Design review of the part built by this model. Coordinates are the model's own, in mm. Round coordinates to 2 decimals unless told otherwise and drop trailing zeros. Loops run counter-clockwise (first coordinate to the right, second up) from the corner with the lowest first, then second, coordinate; pieces in that order, holes last. Notation, with made-up numbers: (46, 34.25) -> (79, 34.25) arc R12 ccw to (79, 50.25) -> close; hole circle Ø6 at (70, -15). An arc over 180 degrees is marked (long way). Use a Markdown table: item, result. Add a question column.
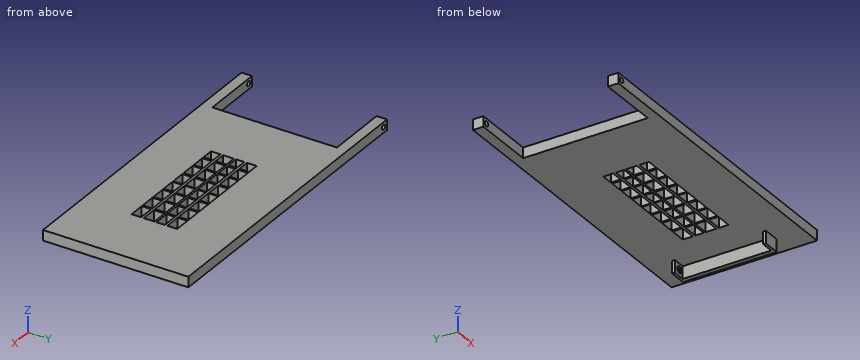
from build123d import *

# Parameters (mm, degrees)
SKETCH1_W               = 600
SKETCH1_H               = 350
BOSS_EXTRUDE1_DEPTH     = 25
SKETCH3_W               = 25
SKETCH3_H               = 25
BOSS_EXTRUDE2_DEPTH     = 150
SKETCH4_R               = 6
CUT_EXTRUDE1_DEPTH      = 370
SKETCH5_W               = 28.359872958
SKETCH5_H               = 23.680958907
SKETCH5_W_2             = 32.02157976
SKETCH5_W_3             = 34.109943658
SKETCH5_W_4             = 34.109943657
SKETCH5_W_5             = 33.413822358
SKETCH5_W_6             = 36.198307555
SKETCH5_W_7             = 38.439491831
SKETCH5_H_2             = 20.187517675
SKETCH5_H_3             = 25.762905436
SKETCH5_H_4             = 22.972002872
CUT_EXTRUDE3_DEPTH      = 30
SKETCH7_W               = 11
SKETCH7_H               = 213.013117536
BOSS_EXTRUDE4_DEPTH     = 30
SKETCH8_W               = 41.071156649
SKETCH8_H               = 6.265091692
BOSS_EXTRUDE5_DEPTH     = 30
SKETCH11_R              = 8
CUT_EXTRUDE6_DEPTH      = 217
CUT_EXTRUDE6_DEPTH_BACK = 4


with BuildPart() as part:
    # Sketch1 → Boss-Extrude1 (new body)
    with BuildSketch(Plane.XY):
        with Locations((300, 175)):
            Rectangle(SKETCH1_W, SKETCH1_H)
    extrude(amount=BOSS_EXTRUDE1_DEPTH)

    # Sketch3 → Boss-Extrude2 (add)
    with BuildSketch(Plane.ZY):
        with Locations((12.5, 12.5)):
            Rectangle(SKETCH3_W, SKETCH3_H)
        with Locations((12.5, 337.5)):
            Rectangle(SKETCH3_W, SKETCH3_H)
    extrude(amount=BOSS_EXTRUDE2_DEPTH)

    # Sketch4 → Cut-Extrude1 (cut)
    with BuildSketch(Plane.XZ):
        with Locations((-137.5, 13.055008402)):
            Circle(SKETCH4_R)
    extrude(amount=-CUT_EXTRUDE1_DEPTH, mode=Mode.SUBTRACT)

    # Sketch5 → Cut-Extrude3 (cut)
    with BuildSketch(Plane.XY.offset(25)):
        with Locations((164.179936479, 215.729513368)):
            Rectangle(SKETCH5_W, SKETCH5_H)
        with Locations((199.243511932, 215.729513368)):
            Rectangle(SKETCH5_W_2, SKETCH5_H)
        with Locations((236.486001436, 215.729513368)):
            Rectangle(SKETCH5_W_3, SKETCH5_H)
        with Locations((275.468794188, 215.729513368)):
            Rectangle(SKETCH5_W_4, SKETCH5_H)
        with Locations((312.015162392, 215.729513368)):
            Rectangle(SKETCH5_W_5, SKETCH5_H)
        with Locations((349.953773195, 215.729513368)):
            Rectangle(SKETCH5_W_3, SKETCH5_H)
        with Locations((389.284626597, 215.729513368)):
            Rectangle(SKETCH5_W_6, SKETCH5_H)
        with Locations((430.780254085, 215.729513368)):
            Rectangle(SKETCH5_W_7, SKETCH5_H)
        with Locations((164.179936479, 187.530183384)):
            Rectangle(SKETCH5_W, SKETCH5_H_2)
        with Locations((199.243511932, 187.530183384)):
            Rectangle(SKETCH5_W_2, SKETCH5_H_2)
        with Locations((236.486001436, 187.530183384)):
            Rectangle(SKETCH5_W_3, SKETCH5_H_2)
        with Locations((275.468794188, 187.530183384)):
            Rectangle(SKETCH5_W_4, SKETCH5_H_2)
        with Locations((312.015162392, 187.530183384)):
            Rectangle(SKETCH5_W_5, SKETCH5_H_2)
        with Locations((349.953773195, 187.530183384)):
            Rectangle(SKETCH5_W_3, SKETCH5_H_2)
        with Locations((389.284626597, 187.530183384)):
            Rectangle(SKETCH5_W_6, SKETCH5_H_2)
        with Locations((430.780254085, 187.530183384)):
            Rectangle(SKETCH5_W_7, SKETCH5_H_2)
        with Locations((430.780254085, 159.688540103)):
            Rectangle(SKETCH5_W_7, SKETCH5_H_3)
        with Locations((389.284626597, 159.688540103)):
            Rectangle(SKETCH5_W_6, SKETCH5_H_3)
        with Locations((349.953773195, 159.688540103)):
            Rectangle(SKETCH5_W_3, SKETCH5_H_3)
        with Locations((312.015162392, 159.688540103)):
            Rectangle(SKETCH5_W_5, SKETCH5_H_3)
        with Locations((275.468794188, 159.688540103)):
            Rectangle(SKETCH5_W_4, SKETCH5_H_3)
        with Locations((236.486001436, 159.688540103)):
            Rectangle(SKETCH5_W_3, SKETCH5_H_3)
        with Locations((199.243511932, 159.688540103)):
            Rectangle(SKETCH5_W_2, SKETCH5_H_3)
        with Locations((164.179936479, 159.688540103)):
            Rectangle(SKETCH5_W, SKETCH5_H_3)
        with Locations((164.179936479, 129.055994257)):
            Rectangle(SKETCH5_W, SKETCH5_H_4)
        with Locations((199.243511932, 129.055994257)):
            Rectangle(SKETCH5_W_2, SKETCH5_H_4)
        with Locations((236.486001436, 129.055994257)):
            Rectangle(SKETCH5_W_3, SKETCH5_H_4)
        with Locations((275.468794188, 129.055994257)):
            Rectangle(SKETCH5_W_4, SKETCH5_H_4)
        with Locations((312.015162392, 129.055994257)):
            Rectangle(SKETCH5_W_5, SKETCH5_H_4)
        with Locations((349.953773195, 129.055994257)):
            Rectangle(SKETCH5_W_3, SKETCH5_H_4)
        with Locations((389.284626597, 129.055994257)):
            Rectangle(SKETCH5_W_6, SKETCH5_H_4)
        with Locations((430.780254085, 129.055994257)):
            Rectangle(SKETCH5_W_7, SKETCH5_H_4)
    extrude(amount=-CUT_EXTRUDE3_DEPTH, mode=Mode.SUBTRACT)

    # Sketch7 → Boss-Extrude4 (add)
    with BuildSketch(Plane(origin=(0, 0, 0), x_dir=(-1, 0, 0), z_dir=(0, 0, -1))):
        with Locations((-545.980889295, 178.828667145)):
            Rectangle(SKETCH7_W, SKETCH7_H)
    extrude(amount=BOSS_EXTRUDE4_DEPTH)

    # Sketch8 → Boss-Extrude5 (add)
    with BuildSketch(Plane(origin=(0, 0, 0), x_dir=(-1, 0, 0), z_dir=(0, 0, -1))):
        with Locations((-530.945310971, 288.467771759)):
            Rectangle(SKETCH8_W, SKETCH8_H)
        with Locations((-530.945310971, 69.189562531)):
            Rectangle(SKETCH8_W, SKETCH8_H)
    extrude(amount=BOSS_EXTRUDE5_DEPTH)

    # Sketch11 → Cut-Extrude6 (cut, two sides)
    with BuildSketch(Plane.XZ.offset(-285.335225913)) as cut_extrude6_sk:
        with Locations((528.139054201, -14.194336347)):
            Circle(SKETCH11_R)
    extrude(amount=CUT_EXTRUDE6_DEPTH, mode=Mode.SUBTRACT)
    extrude(cut_extrude6_sk.sketch, amount=-CUT_EXTRUDE6_DEPTH_BACK, mode=Mode.SUBTRACT)


solid = part.part
1. Insertion check: P1, Ø4, axis at x = 424.5, y = 195, coming from the -Z side; P2, Ø5, axis at x = 530, z = -11, coming from the +Y side; P3, Ø3, axis at y = 146.5, z = -0.5, coming from the -X side. Each pin has a flat end and moves straight along its axis. Give the tip position at first contact, or say it passes through.
2. Consider section A-A on x = 205.5. State the section outline as (y, z) points, plus the area to 3 significant figures.
3. Consider section C-C on x = -13.5. State the section outline as (y, z) points.
4. To check wall thickness, follow probe 1 along Y at (x, z) = (-31.5, 17); probe 2 along Y at (x, z) = (312.5, 2.5); probe 3 along Z at (x, y) = (-137.5, 336.25) (3 decimals). State the ranges of each line that lie inside material, in increasing order. Write a range as from..to.
5. Consider section B-B on y = 252. State the section outline as (x, z) points, plus the area to 3 significant figures.
Verdict:
| question | item | result |
|---|---|---|
| 1 | P1 | passes through |
| 1 | P2 | stops at y = 291.6 |
| 1 | P3 | stops at x = 0 |
| 2 | outline | (0, 0) -> (117.57, 0) -> (117.57, 25) -> (0, 25) -> close; (140.54, 0) -> (146.81, 0) -> (146.81, 25) -> (140.54, 25) -> close; (172.57, 0) -> (177.44, 0) -> (177.44, 25) -> (172.57, 25) -> close; (197.62, 0) -> (203.89, 0) -> (203.89, 25) -> (197.62, 25) -> close; (227.57, 0) -> (350, 0) -> (350, 25) -> (227.57, 25) -> close |
| 2 | area | 6,430 mm² |
| 3 | outline | (0, 0) -> (25, 0) -> (25, 25) -> (0, 25) -> close; (325, 0) -> (350, 0) -> (350, 25) -> (325, 25) -> close |
| 4 | probe 1 | y = 0..25, 325..350 |
| 4 | probe 2 | y = 0..117.57, 140.54..146.81, 172.57..177.44, 197.62..203.89, 227.57..350 |
| 4 | probe 3 | z = 0..7.055, 19.055..25 |
| 5 | outline | (0, 0) -> (540.48, 0) -> (540.48, -30) -> (551.48, -30) -> (551.48, 0) -> (600, 0) -> (600, 25) -> (0, 25) -> close |
| 5 | area | 15,300 mm² |
